from build123d import *

# Parameters (mm, degrees)
BOSS_EXTRUDE1_DEPTH = 1.5
BOSS_EXTRUDE2_DEPTH = 5
BOSS_EXTRUDE3_START = 5
BOSS_EXTRUDE3_DEPTH = 1.5
FILLET1_R           = 5
FILLET2_R           = 1


with BuildPart() as part:
    # Sketch1 → Boss-Extrude1 (new body)
    with BuildSketch(Plane.XY):
        Polygon((0, 40), (0, 32.5), (65.5, 39), (65.5, 40), align=None)
        Polygon((0, 32.5), (0, 27.5), (65.5, 21), (65.5, 39), align=None)
        Polygon((0, 27.5), (0, 12.5), (65.5, 19), (65.5, 21), align=None)
        Polygon((0, 12.5), (0, 7.5), (65.5, 1), (65.5, 19), align=None)
        Polygon((0, 7.5), (0, 0), (65.5, 0), (65.5, 1), align=None)
    extrude(amount=-BOSS_EXTRUDE1_DEPTH)

    # Sketch1_3 → Boss-Extrude2 (add)
    with BuildSketch(Plane.XY):
        Polygon((0, 40), (0, 32.5), (65.5, 39), (65.5, 40), align=None)
        Polygon((0, 27.5), (0, 12.5), (65.5, 19), (65.5, 21), align=None)
        Polygon((0, 7.5), (0, 0), (65.5, 0), (65.5, 1), align=None)
    extrude(amount=BOSS_EXTRUDE2_DEPTH)

    # Sketch1_5 → Boss-Extrude3 (add)
    with BuildSketch(Plane.XY.offset(BOSS_EXTRUDE3_START)):
        Polygon((0, 40), (0, 32.5), (65.5, 39), (65.5, 40), align=None)
        Polygon((0, 32.5), (0, 27.5), (65.5, 21), (65.5, 39), align=None)
        Polygon((0, 27.5), (0, 12.5), (65.5, 19), (65.5, 21), align=None)
        Polygon((0, 12.5), (0, 7.5), (65.5, 1), (65.5, 19), align=None)
        Polygon((0, 7.5), (0, 0), (65.5, 0), (65.5, 1), align=None)
    extrude(amount=BOSS_EXTRUDE3_DEPTH)

    # Fillet1
    fillet1_edges = [part.edges().sort_by_distance(p)[0] for p in [
        (0, 40, 2.5),
        (0, 0, 2.5),
    ]]
    fillet(fillet1_edges, radius=FILLET1_R)

    # Fillet2
    fillet2_edges = [part.edges().sort_by_distance(p)[0] for p in [
        (65.5, 21, 2.5),
        (65.5, 19, 2.5),
    ]]
    fillet(fillet2_edges, radius=FILLET2_R)


solid = part.part
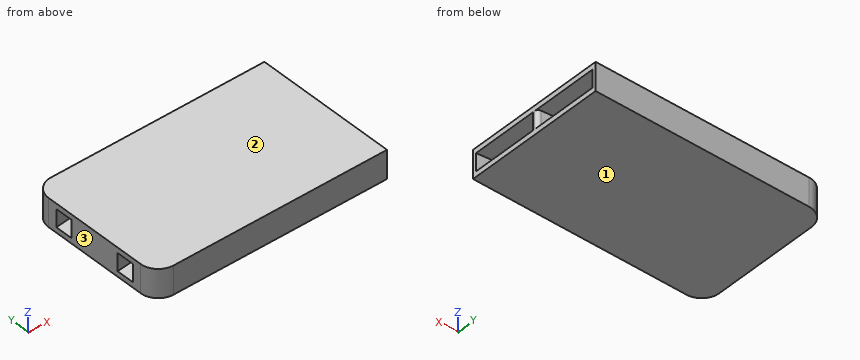
Read the model definition and answer for the solid it produces. Units are mm, in the model's axes. Face numbers are marked on the shaded views. Coordinates: 2 decimals unless noted, no trailing zeros. Order: outer loops, then holes, each group sorted by start corner. A loop starts at its lowest first (then second) coordinate and runs counter-clockwise, first axis right, second up. Notation, with made-up numbers: (-14.75, 30) - (1.25, 30) arc R11 cw to (1.25, 34) - close; hole circle Ø4 at (-8, 63.5). An arc over 180 degrees is marked (long way). Use one line per item in the form item = value.
(1) For a pull along Z with two mould halves and no side action, classify the marked faces 1, 2 and 3 as pulls with the +Z half, pulls with the -Z half, needs draft (parallel to the pull), parting line crosses it, or undercut.
Computed values:
face_1 = pulls with the -Z half
face_2 = pulls with the +Z half
face_3 = needs draft
(2) Section B-B, the plane y = 9 is taken. Give the vertices of the cut face in (x, z).
Computed values:
outline = (0, -1.5) - (65.5, -1.5) - (65.5, 0) - (0, 0) - close; (0, 5) - (65.5, 5) - (65.5, 6.5) - (0, 6.5) - close
(3) Section C-C, the plane x = 12 is taken. Give the vertices of the cut face in (y, z).
Computed values:
outline = (0, -1.5) - (40, -1.5) - (40, 6.5) - (0, 6.5) - close; hole (6.31, 0) - (13.69, 0) - (13.69, 5) - (6.31, 5) - close; hole (26.31, 0) - (33.69, 0) - (33.69, 5) - (26.31, 5) - close
(4) Section D-D, the plane y = 4 is taken. Give the vertices of the cut face in (x, z).
Computed values:
outline = (0.1, -1.5) - (65.5, -1.5) - (65.5, 0) - (35.27, 0) - (35.27, 5) - (65.5, 5) - (65.5, 6.5) - (0.1, 6.5) - close
(5) Section A-A, the plane z = 3 is taken. Give the vertices of the cut face in (x, y), then the cut area to 3 significant figures.
Computed values:
outline = (0, 5) arc R5 ccw to (5, 0) - (65.5, 0) - (65.5, 1) - (0, 7.5) - close; (0, 12.5) - (64.6, 18.91) arc R1 ccw to (65.5, 19.91) - (65.5, 20.09) arc R1 ccw to (64.6, 21.09) - (0, 27.5) - close; (0, 32.5) - (65.5, 39) - (65.5, 40) - (5, 40) arc R5 ccw to (0, 35) - close
area = 1,100 mm²
(6) Straight lines are drawn through the part: L1, parallel to Z at x = 9, y = 33; L2, parallel to Y at x = 23.5, z = 3.25; L3, parallel to Y at x = 11.5, z = 4. For each, find the intervals that lie inside material, in ascending order.
Computed values:
L1 = -1.5 to 0, 5 to 6.5
L2 = 0 to 5.17, 14.83 to 25.17, 34.83 to 40
L3 = 0 to 6.36, 13.64 to 26.36, 33.64 to 40
